```python
from build123d import *

# Parameters (mm, degrees)
BOSS_EXTRUDE1_DEPTH       = 5
F_8_CLEARANCE_HOLE1_D     = 4.4958
F_8_CLEARANCE_HOLE1_DEPTH = 17
F_8_CLEARANCE_HOLE1_TIP   = 1.350674586
SKETCH3_W                 = 6
SKETCH3_H                 = 6
BOSS_EXTRUDE2_DEPTH       = 15
F_8_CLEARANCE_HOLE2_D     = 4.4958
F_8_CLEARANCE_HOLE2_DEPTH = 17
F_8_CLEARANCE_HOLE2_TIP   = 1.350674586


with BuildPart() as part:
    # Sketch1 → Boss-Extrude1 (new body)
    with BuildSketch(Plane(origin=(0, 0, 0), x_dir=(1, 0, 0), z_dir=(0, 1, 0))):
        Polygon((-14.338976611, 0), (30.661023389, 0), (30.661023389, 55.621488653), (8.161023389, 55.621488653), (-14.338976611, 55.621488653), align=None)
    extrude(amount=BOSS_EXTRUDE1_DEPTH)

    # #8 Clearance Hole1
    with Locations(Plane(origin=(22.377803879, 0, -10), x_dir=(0, 0, -1), z_dir=(0, -1, 0))):
        with Locations((0, 0), (0, -27.25), (30.001031232, -13.625)):
            Hole(F_8_CLEARANCE_HOLE1_D / 2, depth=F_8_CLEARANCE_HOLE1_DEPTH)
            with Locations((0, 0, -(F_8_CLEARANCE_HOLE1_DEPTH + F_8_CLEARANCE_HOLE1_TIP / 2))):  # 118° drill point
                Cone(0, F_8_CLEARANCE_HOLE1_D / 2, F_8_CLEARANCE_HOLE1_TIP, mode=Mode.SUBTRACT)

    # Sketch3 → Boss-Extrude2 (add)
    with BuildSketch(Plane(origin=(0, 0, 0), x_dir=(-1, 0, 0), z_dir=(0, -1, 0))):
        with Locations((-8.161023389, 47.5)):
            Rectangle(SKETCH3_W, SKETCH3_H)
        with Locations((-8.161023389, 13)):
            Rectangle(SKETCH3_W, SKETCH3_H)
    extrude(amount=BOSS_EXTRUDE2_DEPTH)

    # #8 Clearance Hole2
    with Locations(Plane(origin=(5.161023389, -11, -47.5), x_dir=(0, 0, -1), z_dir=(-1, 0, 0))):
        with Locations((0, 0), (-34.5, 0)):
            Hole(F_8_CLEARANCE_HOLE2_D / 2, depth=F_8_CLEARANCE_HOLE2_DEPTH)
            with Locations((0, 0, -(F_8_CLEARANCE_HOLE2_DEPTH + F_8_CLEARANCE_HOLE2_TIP / 2))):  # 118° drill point
                Cone(0, F_8_CLEARANCE_HOLE2_D / 2, F_8_CLEARANCE_HOLE2_TIP, mode=Mode.SUBTRACT)


solid = part.part
```
Check sheet for the modelled part. Datum: model origin and axes. Units: mm. A direction names the side the tool comes from. Coordinates: 2 decimals unless noted, no trailing zeros. Write each loop counter-clockwise with the first axis right and the second up, starting at its lowest first coordinate (ties: lowest second). Pieces come first, ordered by that corner, then holes. Notation, with made-up numbers: M 39.5,51 L 89.5,51 A14 cw 89.5,59 Z; hole C -38,2 d3. An arc over 180 degrees is marked long. Write item = value, one per line. Start each with the question number.
1. Sectioned sample at D-D (z = -40). Record the cut outline in (x, y).
2. Sectioned sample at B-B (y = -11). Record the cut outline in (x, z), then the cut area to 3 significant figures.
3. Thickness scan on probe 1 along X at (y, z) = (3.8, -10); probe 2 along Z at (x, y) = (9.55, -11); probe 3 along Z at (x, y) = (7.5, -13.75). Record the ranges inside material, lowest first.
4. Go/stop test with flat-tipped pins: pin 1 (5 mm diameter, centred on y = -11, z = -47.5, fed in from -X); pin 2 (4 mm diameter, centred on x = 22.38, z = -10, fed in from -Y); pin 3 (5 mm diameter, centred on x = 8.75, z = -40, fed in from -Y); pin 4 (6.5 mm diameter, centred on x = 9.5, y = -5, fed in from +Z). Record where each tip stops, or that it passes through.
5. Tool access check on faces 5 (the flat face through (5.161, -7, -47)), 6 (the cylindrical face through (23.053, 2.535, -7.856)), 7 (the flat face through (11.161, -7, -47)), 8 (the flat face through (8, -7, -16)), 9 (the flat face through (8, -7, -50.5)). Record the directions out of +Z, -Z, +X, -X, +Y, -Y that give a thin tool (end or side, any length) a straight path to the whole face; none if there is none.
6. Sectioned sample at C-C (z = -47.5). Record the cut outline in (x, y), then the cut area to 3 significant figures.
7. Sectioned sample at A-A (y = -8). Record the cut outline in (x, z).
8. Mould release check, pull along Z, two halves, no side actions. Record for faces 1 (the flat face through (8, -7, -10)), 2 (the cylindrical face through (10.27, 2.54, -41.66)), 3 (the cylindrical face through (-4.197, 2.535, -7.856)), 4 (the flat face through (11.161, -7, -13)): pulls with the +Z half, pulls with the -Z half, needs draft (parallel to the pull), parting line crosses it, or undercut.
The answers:
q1.outline = M -14.34,0 L 6.5,0 L 6.5,5 L -14.34,5 Z; M 11,0 L 30.66,0 L 30.66,5 L 11,5 Z
q2.outline = M 5.16,-50.5 L 11.16,-50.5 L 11.16,-49.75 L 5.16,-49.75 Z; M 5.16,-45.25 L 11.16,-45.25 L 11.16,-44.5 L 5.16,-44.5 Z; M 5.16,-16 L 11.16,-16 L 11.16,-15.25 L 5.16,-15.25 Z; M 5.16,-10.75 L 11.16,-10.75 L 11.16,-10 L 5.16,-10 Z
q2.area = 18.1 mm²
q3.probe_1 = -14.34 to -7.12, -2.62 to 20.13, 24.63 to 30.66
q3.probe_2 = -50.5 to -49.75, -45.25 to -44.5, -16 to -15.25, -10.75 to -10
q3.probe_3 = -50.5 to -44.5, -16 to -10
q4.pin_1 = 5.16
q4.pin_2 = through
q4.pin_3 = 0
q4.pin_4 = -10
q5.face_5 = +Z, -Z, -X, -Y
q5.face_6 = +Y, -Y
q5.face_7 = +Z, -Z, +X, -Y
q5.face_8 = +X, -X, -Y
q5.face_9 = -Z, +X, -X, -Y
q6.outline = M -14.34,0 L 5.16,0 L 5.16,-8.75 L 11.16,-8.75 L 11.16,0 L 30.66,0 L 30.66,5 L -14.34,5 Z; M 5.16,-15 L 11.16,-15 L 11.16,-13.25 L 5.16,-13.25 Z
q6.area = 288 mm²
q7.outline = M 5.16,-50.5 L 11.16,-50.5 L 11.16,-44.5 L 5.16,-44.5 Z; M 5.16,-16 L 11.16,-16 L 11.16,-10 L 5.16,-10 Z
q8.face_1 = pulls with the +Z half
q8.face_2 = undercut
q8.face_3 = undercut
q8.face_4 = needs draft
